Design review of the part shown in the three views and the two pictorial views. Dimensions are in mm from the part's minimum x, y and z. Give positions to 0.01 mm unless a question says otherwise; leave off trailing zeros. Order: outer loops, then holes, each group sorted by start corner. A loop starts at its lowest first (then second) coordinate and runs counter-clockwise, first axis right, second up.
Item 1: Consider section C-C (x = 2.25). Give the boundary of the cut face in (y, z).
Item 2: For probe 1 along Z at (x, y) = (3.25, 0.75) (1 decimal); probe 2 along Z at (x, y) = (6.5, 1.25) (1 decimal); probe 3 along X at (y, z) = (1, 4.5) (1 decimal), list the stretches that pass through material, from the lowest coordinate up.
Item 3: Consider section B-B (y = 0.8). Give the boundary of the cut face in (x, z) (1 decimal).
Item 4: The part is to be moulded in two halves that separate along Y. For the marked faces 1 and 2, say which applies: released by +Y, released by -Y, zero draft, split by the parting line, or undercut.
Item 5: Consider section A-A (x = 4.5). Give the boundary of the cut face in (y, z).
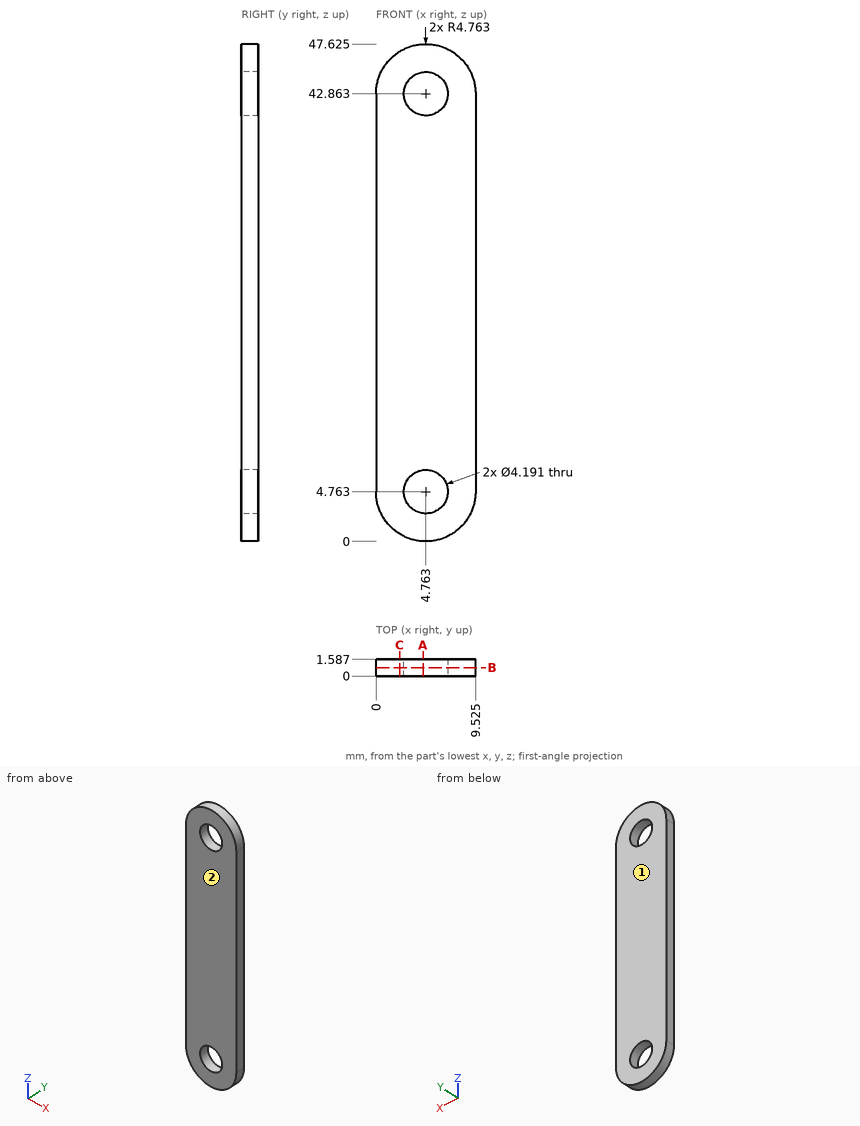
Resolved:
1. outline: (0, 0.72) - (1.59, 0.72) - (1.59, 46.91) - (0, 46.91) - close
2. probe 1: z = 0.2 to 3.3, 6.2 to 41.4, 44.3 to 47.4
2. probe 2: z = 0.3 to 3.6, 5.9 to 41.7, 44 to 47.3
2. probe 3: x = 0 to 2.7, 6.8 to 9.5
3. outline: (0, 4.8) arc R4.8 ccw to (9.5, 4.8) - (9.5, 42.9) arc R4.8 ccw to (0, 42.9) - close; hole circle Ø4.2 at (4.8, 4.8); hole circle Ø4.2 at (4.8, 42.9)
4. face 1: released by +Y
4. face 2: released by -Y
5. outline: (0, 0.01) - (1.59, 0.01) - (1.59, 2.68) - (0, 2.68) - close; (0, 6.84) - (1.59, 6.84) - (1.59, 40.78) - (0, 40.78) - close; (0, 44.94) - (1.59, 44.94) - (1.59, 47.62) - (0, 47.62) - close
